```python
from build123d import *

# Parameters (mm, degrees)
BOSS_EXTRUDE1_DEPTH = 4
SKETCH2_R           = 3
CUT_EXTRUDE3_DEPTH  = 170.752761391
BOSS_EXTRUDE3_DEPTH = 6.35
CHAMFER1_SIZE       = 8.660254038
CHAMFER1_SIZE_2     = 15
BOSS_EXTRUDE4_START = 6.35
SKETCH8_R           = 3
BOSS_EXTRUDE4_DEPTH = 6.35
SKETCH9_W           = 4
SKETCH9_H           = 18
BOSS_EXTRUDE5_DEPTH = 15.875
SKETCH10_R          = 3
CUT_EXTRUDE4_DEPTH  = 110.875
FILLET3_R           = 5
SKETCH11_R          = 5
CUT_EXTRUDE5_DEPTH  = 15.875
FILLET4_R           = 2


with BuildPart() as part:
    # Sketch1 → Boss-Extrude1 (new body)
    with BuildSketch(Plane(origin=(0, 0, 0), x_dir=(1, 0, 0), z_dir=(0, 1, 0))):
        Polygon((0, 0), (120, 0), (120, -50), (4, -117.666666667), (4, -120), (0, -120), align=None)
    extrude(amount=BOSS_EXTRUDE1_DEPTH)

    # Sketch2 → Cut-Extrude3 (cut, through all)
    with BuildSketch(Plane(origin=(0, 4, 0), x_dir=(1, 0, 0), z_dir=(0, 1, 0))):
        with Locations(Location((112, -8, 0), (0, 0, 270))):
            Circle(SKETCH2_R)
        with Locations(Location((112, -43, 0), (0, 0, 270))):
            Circle(SKETCH2_R)
        Polygon((104, -8), (104, -50.071704007), (8, -106.071704007), (8, -8), align=None)
    extrude(amount=-CUT_EXTRUDE3_DEPTH, mode=Mode.SUBTRACT)

    # Sketch7 → Boss-Extrude3 (add)
    with BuildSketch(Plane(origin=(0, 4, 0), x_dir=(1, 0, 0), z_dir=(0, 1, 0))):
        Polygon((118, -48.851259335), (2.992257949, -115.939108865), (4, -117.666666667), (120, -50), (120, 0), (2.992257949, 0), (2.992257949, -2), (118, -2), align=None)
    extrude(amount=BOSS_EXTRUDE3_DEPTH)

    # Chamfer1
    # the kernel refuses this chamfer: 15, 8.660254038 mm, written as the material it takes off along each edge
    with BuildSketch(Plane(origin=(-16.561105336, 10.35, 82.41905752), x_dir=(0, -1, 0), z_dir=(0.5038710255240854, 0, 0.863778900898434))) as chamfer1_piece_1_section:
        Polygon((CHAMFER1_SIZE, 0), (0, CHAMFER1_SIZE_2), (0, 0), align=None)
    chamfer1_piece_1 = extrude(amount=79.612572639, mode=Mode.PRIVATE)
    chamfer1_piece_1 = split(chamfer1_piece_1, bisect_by=Plane(origin=(-16.561105336, 4, 82.41905752), z_dir=(0, 1, 0)), keep=Keep.TOP, mode=Mode.PRIVATE)
    add(chamfer1_piece_1, mode=Mode.SUBTRACT)

    # Sketch8 → Boss-Extrude4 (add)
    # profile 1 of 2: a face of its own
    with BuildSketch(Plane(origin=(0, 4, 0), x_dir=(1, 0, 0), z_dir=(0, 1, 0)).offset(BOSS_EXTRUDE4_START)):
        with BuildLine():
            Line((112, -14.5), (118, -14.5))
            Line((118, -14.5), (118, -2))
            Line((118, -2), (105.5, -2))
            Line((105.5, -2), (105.5, -8))
            ThreePointArc((105.5, -8), (107.403805922, -12.596194078), (112, -14.5))
        make_face()
        with Locations(Location((112, -8, 0), (0, 0, 270))):
            Circle(SKETCH8_R, mode=Mode.SUBTRACT)
    # profile 2 of 2: a face of its own
    with BuildSketch(Plane(origin=(0, 4, 0), x_dir=(1, 0, 0), z_dir=(0, 1, 0)).offset(BOSS_EXTRUDE4_START)):
        with BuildLine():
            Line((112, -36.5), (118, -36.5))
            Line((118, -36.5), (118, -48.851259335))
            Line((118, -48.851259335), (105.5, -56.142926002))
            Line((105.5, -56.142926002), (105.5, -43))
            ThreePointArc((105.5, -43), (107.403805922, -38.403805922), (112, -36.5))
        make_face()
        with Locations(Location((112, -43, 0), (0, 0, 270))):
            Circle(SKETCH8_R, mode=Mode.SUBTRACT)
    extrude(amount=-BOSS_EXTRUDE4_DEPTH)

    # Sketch9 → Boss-Extrude5 (add)
    with BuildSketch(Plane(origin=(0, 4, 0), x_dir=(1, 0, 0), z_dir=(0, 1, 0))):
        with Locations((2, -9)):
            Rectangle(SKETCH9_W, SKETCH9_H)
        with Locations((2, -111)):
            Rectangle(SKETCH9_W, SKETCH9_H)
    extrude(amount=BOSS_EXTRUDE5_DEPTH)

    # Sketch10 → Cut-Extrude4 (cut)
    with BuildSketch(Plane(origin=(4, 0, 0), x_dir=(0, 0, -1), z_dir=(1, 0, 0))):
        with Locations((-9, 11.9375)):
            Circle(SKETCH10_R)
        with Locations((-111, 11.9375)):
            Circle(SKETCH10_R)
    extrude(amount=-CUT_EXTRUDE4_DEPTH, mode=Mode.SUBTRACT)

    # Fillet3
    # the kernel refuses this fillet: 5 mm, written as the material it adds along each edge
    with BuildSketch(Plane(origin=(105.5, 10.35, 56.142926002), x_dir=(-0.863778900898437, 0, 0.50387102552408), z_dir=(0, -1, 0))) as fillet3_piece_1:
        with BuildLine():
            CenterArc((FILLET3_R * 0.574370332454, FILLET3_R), FILLET3_R, 210.256437164, 59.743562836)
            Line((-FILLET3_R * 0.289408568444, FILLET3_R * 0.496128974476), (0, 0))
            Line((0, 0), (FILLET3_R * 0.574370332454, 0))
        make_face()
    extrude(amount=6.35)
    with BuildSketch(Plane(origin=(118, 10.35, 36.5), x_dir=(-1, 0, 0), z_dir=(0, -1, 0))) as fillet3_piece_2:
        with BuildLine():
            CenterArc((FILLET3_R, FILLET3_R), FILLET3_R, 180, 90)
            Line((0, FILLET3_R), (0, 0))
            Line((0, 0), (FILLET3_R, 0))
        make_face()
    extrude(amount=6.35)
    with BuildSketch(Plane(origin=(118, 10.35, 14.5), x_dir=(-1, 0, 0), z_dir=(0, -1, 0)), Plane(origin=(105.5, 10.35, 2), x_dir=(-1, 0, 0), z_dir=(0, -1, 0))) as fillet3_piece_3:
        with BuildLine():
            CenterArc((FILLET3_R, -FILLET3_R), FILLET3_R, 90, 90)
            Line((0, -FILLET3_R), (0, 0))
            Line((0, 0), (FILLET3_R, 0))
        make_face()
    extrude(amount=6.35)
    with BuildSketch(Plane(origin=(4, 0, 117.666666667), x_dir=(0.863778900898435, 0, -0.5038710255240835), z_dir=(0, 1, 0))) as fillet3_piece_4:
        with BuildLine():
            CenterArc((2.835867325, -5), FILLET3_R, 90, 53.351575298)
            Line((-1.17569906, -2.015484102), (0, 0))
            Line((0, 0), (2.835867325, 0))
        make_face()
    extrude(amount=4)
    with BuildSketch(Plane(origin=(8, 4, 106.071704007), x_dir=(0.8637789008984339, 0, -0.5038710255240852), z_dir=(0, -1, 0))) as fillet3_piece_5:
        with BuildLine():
            CenterArc((FILLET3_R * 1.74103699912, -FILLET3_R), FILLET3_R, 90, 120.256437164)
            Line((FILLET3_R * 0.877258098222, -FILLET3_R * 1.50387102552), (0, 0))
            Line((0, 0), (FILLET3_R * 1.74103699912, 0))
        make_face()
    extrude(amount=4)
    with BuildSketch(Plane(origin=(104, 4, 50.071704007), x_dir=(-0.8637789008984337, 0, 0.5038710255240859), z_dir=(0, -1, 0))) as fillet3_piece_6:
        with BuildLine():
            CenterArc((FILLET3_R * 0.574370332454, FILLET3_R), FILLET3_R, 210.256437164, 59.743562836)
            Line((-FILLET3_R * 0.289408568444, FILLET3_R * 0.496128974476), (0, 0))
            Line((0, 0), (FILLET3_R * 0.574370332454, 0))
        make_face()
    extrude(amount=4)
    with BuildSketch(Plane(origin=(104, 4, 8), x_dir=(-1, 0, 0), z_dir=(0, -1, 0)), Plane(origin=(8, 4, 8), x_dir=(0, 0, 1), z_dir=(0, -1, 0))) as fillet3_piece_7:
        with BuildLine():
            CenterArc((FILLET3_R, -FILLET3_R), FILLET3_R, 90, 90)
            Line((0, -FILLET3_R), (0, 0))
            Line((0, 0), (FILLET3_R, 0))
        make_face()
    extrude(amount=4)
    with BuildSketch(Plane(origin=(4, 4, 102), x_dir=(0, 1, 0), z_dir=(-1, 0, 0)), Plane(origin=(4, 4, 18), x_dir=(0, 0, 1), z_dir=(-1, 0, 0))) as fillet3_piece_8:
        with BuildLine():
            CenterArc((FILLET3_R, FILLET3_R), FILLET3_R, 180, 90)
            Line((0, FILLET3_R), (0, 0))
            Line((0, 0), (FILLET3_R, 0))
        make_face()
    extrude(amount=4)
    # the kernel refuses this fillet: 5 mm, written as the material it takes off along each edge
    with BuildSketch(Plane(origin=(120, 22.85, 0), x_dir=(-1, 0, 0), z_dir=(0, -1, 0))) as fillet3_2_piece_1:
        with BuildLine():
            CenterArc((FILLET3_R, -FILLET3_R), FILLET3_R, 90, 90)
            Line((0, -FILLET3_R), (0, 0))
            Line((0, 0), (FILLET3_R, 0))
        make_face()
    extrude(amount=35.35, mode=Mode.SUBTRACT)
    with BuildSketch(Plane(origin=(120, 17.529629156, 50), x_dir=(0, 0, -1), z_dir=(0, -1, 0))) as fillet3_2_piece_2:
        with BuildLine():
            CenterArc((FILLET3_R * 0.574370332454, -FILLET3_R), FILLET3_R, 90, 59.743562836)
            Line((-FILLET3_R * 0.289408568444, -FILLET3_R * 0.496128974476), (0, 0))
            Line((0, 0), (FILLET3_R * 0.574370332454, 0))
        make_face()
    extrude(amount=24.709258311, mode=Mode.SUBTRACT)
    with BuildSketch(Plane(origin=(-12.5, 19.875, 120), x_dir=(0, 0, -1), z_dir=(1, 0, 0)), Plane(origin=(-12.5, 19.875, 0), x_dir=(0, -1, 0), z_dir=(1, 0, 0)), Plane(origin=(16.5, 19.875, 18), x_dir=(0, -1, 0), z_dir=(-1, 0, 0))) as fillet3_2_piece_3:
        with BuildLine():
            CenterArc((FILLET3_R, -FILLET3_R), FILLET3_R, 90, 90)
            Line((0, -FILLET3_R), (0, 0))
            Line((0, 0), (FILLET3_R, 0))
        make_face()
    extrude(amount=29, mode=Mode.SUBTRACT)
    with BuildSketch(Plane(origin=(16.5, 19.875, 102), x_dir=(0, -1, 0), z_dir=(-1, 0, 0))) as fillet3_2_piece_4:
        with BuildLine():
            CenterArc((FILLET3_R, FILLET3_R), FILLET3_R, 180, 90)
            Line((0, FILLET3_R), (0, 0))
            Line((0, 0), (FILLET3_R, 0))
        make_face()
    extrude(amount=29, mode=Mode.SUBTRACT)

    # Sketch11 → Cut-Extrude5 (cut)
    with BuildSketch(Plane(origin=(0, 4, 0), x_dir=(1, 0, 0), z_dir=(0, 1, 0))):
        with Locations(Location((112, -25.5, 0), (0, 0, 270))):
            Circle(SKETCH11_R)
    extrude(amount=-CUT_EXTRUDE5_DEPTH, mode=Mode.SUBTRACT)

    # Fillet4
    fillet4_edges = [part.edges().sort_by_distance(p)[0] for p in [
        (4, 7.175, 2),
    ]]
    fillet(fillet4_edges, radius=FILLET4_R)


solid = part.part
```
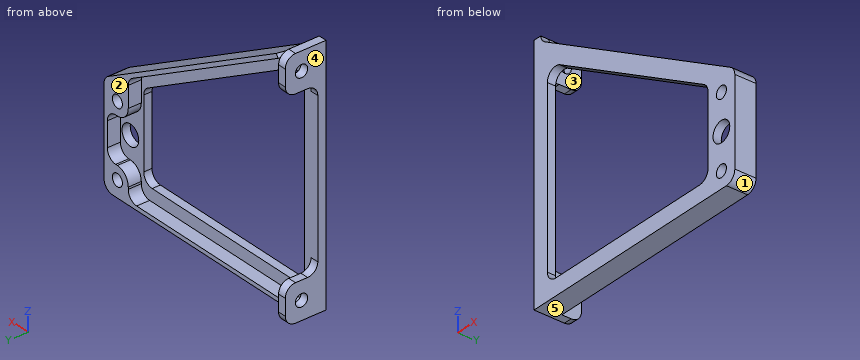
Can you work these out from the model? Positions are in its coordinate system, mm. Face numbers are marked on the shaded views. A direction names the side the tool comes from. Coordinates: 2 decimals unless noted, no trailing zeros. Write each loop counter-clockwise with the first axis right and the second up, starting at its lowest first coordinate (ties: lowest second). Pieces come first, ordered by that corner, then holes. Notation, with made-up numbers: (20, -7) - (40, -7) arc R14 ccw to (40, -1) - close; hole circle Ø3 at (-40, 54.25). An arc over 180 degrees is marked (long way). Return JSON: item names as keys, results as strings.
Q1. If we section it at A-A (y = 1.5): Please give me the cut outline in (x, z).
Computed values:
{"outline": "(0, 0) - (115, 0) arc R5 ccw to (120, 5) - (120, 47.13) arc R5 ccw to (117.52, 51.45) - (6.45, 116.24) arc R5 cw to (4, 120) - (0, 120) - close; hole (8, 13) arc R5 ccw to (13, 8) - (99, 8) arc R5 ccw to (104, 13) - (104, 47.2) arc R5 ccw to (101.52, 51.52) - (15.52, 101.69) arc R5 ccw to (8, 97.37) - close; hole circle Ø10 at (112, 25.5); hole circle Ø6 at (112, 8); hole circle Ø6 at (112, 43)"}
Q2. Thinking about a two-plate mould opening in X: for the marked faces 3, 4 and 5, which applies, +X half, -X half, draft (parallel to the pull), parting line (faces both ways), or undercut?
Computed values:
{"face 3": "undercut", "face 4": "-X half", "face 5": "draft"}
Q3. If we section it at B-B (z = 78.5): Please give me the cut outline in (x, y).
Computed values:
{"outline": "(0, 0) - (8, 0) - (8, 4) - (0, 4) - close; (55.27, 0) - (71.14, 0) - (71.14, 10.35) - (67.17, 10.35) - (67.17, 4) - (55.27, 4) - close"}
Q4. If we section it at C-C (x = 68.5): Please give me the cut outline in (y, z).
Computed values:
{"outline": "(0, 0) - (10.35, 0) - (10.35, 2) - (4, 2) - (4, 8) - (0, 8) - close; (0, 70.78) - (4, 70.78) - (4, 77.73) - (10.35, 77.73) - (10.35, 80.04) - (0, 80.04) - close"}
Q5. Please list where these lines run through material, in increasing order: L1, parallel to X at y = 7.75, z = 8; L2, parallel to Y at x = 2, z = 111 (1 decimal); L3, parallel to X at y = 7.25, z = 43. Write a range as from..to.
Computed values:
{"L1": "x = 0..4, 105.5..109, 115..120", "L2": "y = 0..8.9, 14.9..19.9", "L3": "x = 105.5..109, 115..120"}
Q6. I'm going to push flat-ended pins straight in: pin 1 Ø1.9 at (y, z) = (6, 25.5) entering from -X; pin 2 Ø2 at (y, z) = (3, 72.5) entering from +X; pin 3 Ø3 at (x, y) = (27, 2.5) entering from +Z (3 decimals). Where does each tip first touch, or does it pass through?
Computed values:
{"pin 1": "stops at x = 118", "pin 2": "stops at x = 83.14", "pin 3": "stops at z = 105.125"}
Q7. On a 3-axis mill with a long thin cutter (end or side, diameter ignored), from which of +Z, -Z, +X, -X, +Y, -Y can I reach the whole of each face in a straight line? I mean the marked faces 1 and 2. Say none if no direction works.
Computed values:
{"face 1": "-Z, +X, +Y, -Y", "face 2": "+Z, -Z, +X, +Y"}
